```python
from build123d import *

# Parameters (mm, degrees)
SLOT_DEPTH      = 20.063575779
SLOT_DEPTH_BACK = 20.063575779
FILLET1_R       = 0.3175


with BuildPart() as part:
    # Sketch2 → Revolve1 (revolve)
    with BuildSketch(Plane(origin=(0, 0, 0), x_dir=(0, 0, -1), z_dir=(1, 0, 0)), mode=Mode.PRIVATE) as revolve1_sk:
        with BuildLine():
            Line((0, 0), (-15.7988, 0))
            Line((-15.7988, 0), (-15.7988, 1.037166667))
            ThreePointArc((-15.7988, 1.037166667), (-13.640498544, 2.570299796), (-11.049, 3.1115))
            Line((-11.049, 3.1115), (-11.049, 2.9464))
            Line((-11.049, 2.9464), (-1.778, 2.9464))
            Line((-1.778, 2.9464), (-1.778, 7.5438))
            Line((-1.778, 7.5438), (0, 7.5438))
            Line((0, 7.5438), (0, 0))
        make_face()
    revolve(revolve1_sk.sketch.rotate(Axis((0, 0, 0), (0, 0, 1)), 90), axis=Axis((0, 0, 0), (0, 0, 1)))

    # Sketch3 → Slot (cut, two sides: drawn at the far end of the back side and taken through both)
    with BuildSketch(Plane(origin=(0, 0, 0), x_dir=(0, 0, -1), z_dir=(1, 0, 0)).offset(-SLOT_DEPTH_BACK)):
        with BuildLine():
            Line((-9.249833333, 0.518583333), (-15.7988, 0.518583333))
            Line((-15.7988, 0.518583333), (-15.7988, -0.518583333))
            Line((-15.7988, -0.518583333), (-9.249833333, -0.518583333))
            ThreePointArc((-9.249833333, -0.518583333), (-8.73125, 0), (-9.249833333, 0.518583333))
        make_face()
    extrude(amount=SLOT_DEPTH + SLOT_DEPTH_BACK, mode=Mode.SUBTRACT)

    # Fillet1
    fillet1_edges = [part.edges().sort_by_distance(p)[0] for p in [
        (7.5438, 0, 0),
    ]]
    fillet(fillet1_edges, radius=FILLET1_R)


solid = part.part
```
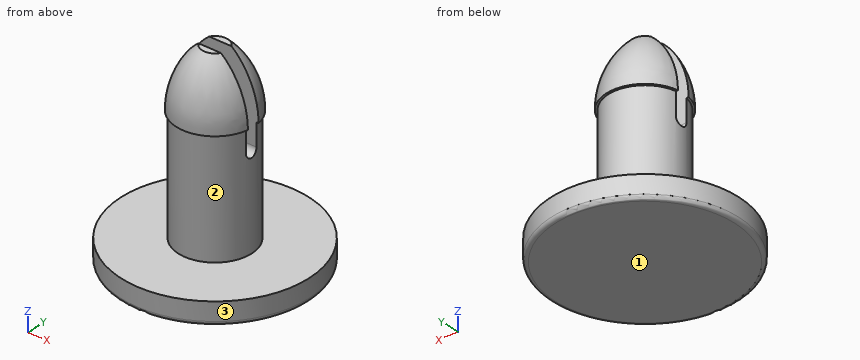
The model under review builds one solid part; all positions refer to its coordinate system, in mm. Face numbers are marked on the shaded views. Round coordinates to 2 decimals unless told otherwise and drop trailing zeros. Loops run counter-clockwise (first coordinate to the right, second up) from the corner with the lowest first, then second, coordinate; pieces in that order, holes last. Notation, with made-up numbers: (38.5, 9) - (44.5, 9) arc R24 ccw to (44.5, 42) - close; hole circle Ø6 at (1.5, 27.25). An arc over 180 degrees is marked (long way). Use a Markdown table: item, result. Add a question column.
Q1. For probe 1 along Y at (x, z) = (-1.5, 9); probe 2 along Y at (x, z) = (-2, 13); probe 3 along Z at (x, y) = (3.25, 4), list the stretches that pass through material, from the lowest coordinate up.
Q2. Insertion check: pin 1 Ø4 at (y, z) = (-4, 5) entering from +X; pin 2 Ø6 at (x, z) = (1, 2) entering from -Y; pin 3 Ø2 at (y, z) = (-4, 10) entering from +X; pin 4 Ø3 at (x, z) = (-0.5, 14) entering from -Y. Each pin has a flat end and moves straight along its axis. Give the tip position at first contact, or say it passes through.
Q3. Add section B-B (z = 2.5). State the section outline as (x, y) points.
Q4. The part is to be moulded in two halves that separate along Z. For the marked faces 1, 2 and 3, say which applies: pulls with the +Z half, pulls with the -Z half, needs draft (parallel to the pull), parting line crosses it, or undercut.
Q5. Add section A-A (y = 0). State the section outline as (x, z) points (1 decimal), plus the area to 3 significant figures.
Worked answers:
| question | item | result |
|---|---|---|
| 1 | probe 1 | -2.54 to -0.45, 0.45 to 2.54 |
| 1 | probe 2 | -1.97 to -0.52, 0.52 to 1.97 |
| 1 | probe 3 | 0 to 1.78 |
| 2 | pin 1 | x = 2.16 |
| 2 | pin 2 | y = -7.54 |
| 2 | pin 3 | through |
| 2 | pin 4 | y = -2.93 |
| 3 | outline | circle Ø5.89 at (0, 0) |
| 4 | face 1 | pulls with the -Z half |
| 4 | face 2 | undercut |
| 4 | face 3 | needs draft |
| 5 | outline | (-7.5, 0.3) arc R0.3 ccw to (-7.2, 0) - (7.2, 0) arc R0.3 ccw to (7.5, 0.3) - (7.5, 1.8) - (2.9, 1.8) - (2.9, 8.7) - (-2.9, 8.7) - (-2.9, 1.8) - (-7.5, 1.8) - close |
| 5 | area | 67.8 mm² |
